Autodesk Inventor part; units mm, degrees
ref_plane "YZ Plane" through (0, 0, 0) normal (1, 0, 0) x (0, 1, 0)
ref_plane "XZ Plane" through (0, 0, 0) normal (0, 1, 0) x (-1, 0, 0)
ref_plane "XY Plane" through (0, 0, 0) normal (0, 0, 1) x (1, 0, 0)
sketch "Sketch1" plane through (0, 0, 0) normal (0, 0, 1) x (1, 0, 0)
  line L0 (0, 158.75) -> (9.525, 158.75)
  line L1 (9.525, 158.75) -> (9.525, 138.1125)
  line L2 (9.525, 138.1125) -> (6.35, 138.1125)
  line L3 (6.35, 138.1125) -> (6.35, 131.7625)
  line L4 (6.35, 131.7625) -> (7.9375, 131.7625)
  line L5 (7.9375, 131.7625) -> (7.9375, 31.75)
  line L6 (7.9375, 31.75) -> (6.35, 31.75)
  line L7 (6.35, 31.75) -> (6.35, 9.6012)
  line L8 (6.35, 9.6012) -> (4.7625, 9.6012)
  line L9 (4.7625, 9.6012) -> (4.7625, 6.35)
  line L10 (4.7625, 6.35) -> (6.35, 6.35)
  line L11 (6.35, 6.35) -> (6.35, 0)
  line L12 (6.35, 0) -> (0, 0)
  line L13 (0, 0) -> (0, 158.75)
  dimension "d0" = 12.7
  dimension "d1" = 9.525
  dimension "d3" = 12.7
  dimension "d4" = 15.875
  dimension "d5" = 12.7
  dimension "d6" = 19.05
  dimension "d7" = 20.6375
  dimension "d8" = 6.35
  dimension "d9" = 100.0125
  dimension "d10" = 6.35
  dimension "d11" = 3.2512
  dimension "d12" = 158.75
revolve "Revolution1" add sketch "Sketch1" angle 360 about axis through (0, 0, 0) along (0, 1, 0)
thread "Thread1"
sketch "Sketch2" plane through (0, 0, 0) normal (0, 0, 1) x (1, 0, 0)
  line L0 (-9.525, 158.75) -> (9.525, 158.75)
  circle A0 centre (0, 148.4313) radius 4.3656
  point P0 (0, 158.75)
  dimension "d16" = 8.7312
  dimension "d17" = 10.3187
extrude "Extrusion1" cut sketch "Sketch2" along normal through all both and the other way through all
fillet "Fillet1" radius 1.5875 1 edges at (-9.525, 158.75, 0)
properties part number "Vise_Screw" material "Steel, Mild"
Can you work these out from the model? Positions are in its coordinate system, mm. A direction names the side the tool comes from. Coordinates: 2 decimals unless noted, no trailing zeros. Write each loop counter-clockwise with the first axis right and the second up, starting at its lowest first coordinate (ties: lowest second). Pieces come first, ordered by that corner, then holes.
Q1. Which directions (+Z, -Z, +X, -X, +Y, -Y) give clear straight access to the entire face, cutting with the end or side of a thin tool? Please do faces 5 (the face through (9.085, 147.504, 2.861)), 6 (the face through (-3.78, 7.95, -2.9)), 7 (the face through (-1.38, 20.52, -6.2)).
Results found:
face 5: +Y, -Y
face 6: none
face 7: -Y
Q2. Imagine slicing it at D-D, the plane y = 92. List the corners of the cut face in (x, z) for me (1 decimal).
Results found:
outline: circle Ø15.9 at (0, 0)
Q3. Please list where these lines run through material, in increasing order: L1, parallel to Y at x = 0, z = -3.75; L2, parallel to Y at x = 0, z = 5.75; L3, parallel to Y at x = -7.5, z = 0.5.
Results found:
L1: y = 0 to 144.07, 152.8 to 158.75
L2: y = 0 to 6.35, 9.6 to 144.07, 152.8 to 158.75
L3: y = 31.75 to 131.76, 138.11 to 158.75
Q4. Imagine slicing it at C-C, the plane y = 12.5. List the corners of the cut face in (x, z) for me.
Results found:
outline: circle Ø12.7 at (0, 0)
Q5. If we mould it in two halves opening along Y, with no side actions, what happens to faces 1 (the face through (0, 0, 0)), 2 (the face through (2.014, 144.558, 0.133)), 3 (the face through (6.2, 138.112, 2)), 4 (the face through (-1.72, 81.06, -7.75))? For each: +Y half, -Y half, draft (parallel to the pull), parting line (faces both ways), or undercut.
Results found:
face 1: -Y half
face 2: undercut
face 3: undercut
face 4: draft
Q6. For P1, Ø8, axis at x = 4, y = 113, coming from the +Z side; P2, Ø5, axis at x = -7, y = 67.5, coming from the -Z side; P3, Ø1, axis at y = 100, z = -4.5, coming from the +X side, each with a flat end and sliding along its axis, tell me the tip position at first contact or that it passes through.
Results found:
P1: stops at z = 7.94
P2: stops at z = -6.54
P3: stops at x = 6.86
